Here's how the part is built. I have some questions about the finished solid (model axes, mm). Face numbers are marked on the shaded views. Coordinates: 2 decimals unless noted, no trailing zeros. Loops run counter-clockwise (first coordinate to the right, second up) from the corner with the lowest first, then second, coordinate; pieces in that order, holes last. Notation, with made-up numbers: (41.25, 38.5) - (48.25, 38.5) arc R22 ccw to (48.25, 55.5) - close; hole circle Ø6 at (53, -36.75). An arc over 180 degrees is marked (long way). Use a Markdown table: item, result.
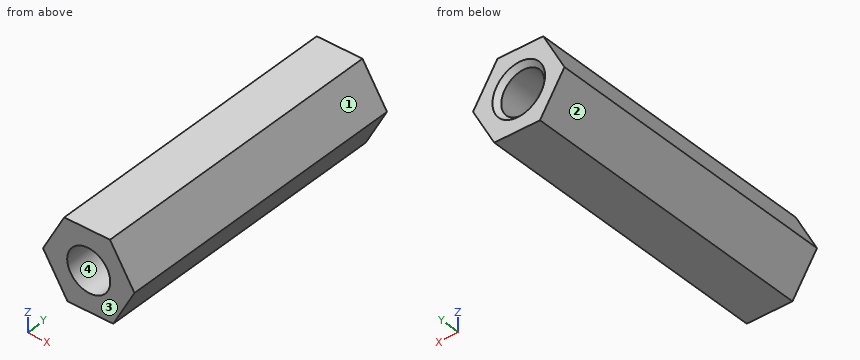
```python
from build123d import *

# Parameters (mm, degrees)
SKETCH_1_R                   = 1.1
EXTRUDE_1_DEPTH              = 17
HOLE_WIZARD_M3_2_D           = 2.5
HOLE_WIZARD_M3_2_CSINK_D     = 3.05
HOLE_WIZARD_M3_2_CSINK_ANGLE = 90


with BuildPart() as part:
    # 草图1 → 凸台-拉伸1 (new body)
    with BuildSketch(Plane(origin=(0, 0, 0), x_dir=(1, 0, 0), z_dir=(0, 1, 0))):
        Polygon((1.231724884, -2.352910356), (2.653542583, -0.109750138), (1.421817699, 2.243160218), (-1.231724884, 2.352910356), (-2.653542583, 0.109750138), (-1.421817699, -2.243160218), align=None)
        Circle(SKETCH_1_R, mode=Mode.SUBTRACT)
    extrude(amount=EXTRUDE_1_DEPTH)

    # M3 螺纹孔2 (through all)
    with Locations(Plane(origin=(0, 17, 0), x_dir=(1, 0, 0), z_dir=(0, 1, 0))):
        with Locations((0, 0)):
            CounterSinkHole(HOLE_WIZARD_M3_2_D / 2, HOLE_WIZARD_M3_2_CSINK_D / 2, counter_sink_angle=HOLE_WIZARD_M3_2_CSINK_ANGLE)


solid = part.part
```
Q1. I want a section at A-A, the plane y = 13.75. Write out the boundary of the cut face in (x, z).
Check values:
| item | result |
|---|---|
| outline | (-2.65, -0.11) - (-1.23, -2.35) - (1.42, -2.24) - (2.65, 0.11) - (1.23, 2.35) - (-1.42, 2.24) - close; hole circle Ø2.5 at (0, 0) |
Q2. I want a section at C-C, the plane z = 1.7. Write out the boundary of the cut face in (x, y), then the cut area to 3 significant figures.
Check values:
| item | result |
|---|---|
| outline | (-1.71, 0) - (1.65, 0) - (1.65, 17) - (-1.71, 17) - close |
| area | 57.0 mm^2 |
Q3. Please list where these lines run through material, in increasing order: L1, parallel to Z at x = 0.6, y = 6; L2, parallel to X at y = 16.25, z = -0.9; L3, parallel to Z at x = 0.2, y = 16.25. Write a range as from..to.
Check values:
| item | result |
|---|---|
| L1 | -2.28..-1.1, 1.1..2.33 |
| L2 | -2.15..-0.87, 0.87..2.12 |
| L3 | -2.29..-1.23, 1.23..2.31 |
Q4. If we mould it in two halves opening along Z, with no side actions, what happens to the marked faces 1, 2, 3 and 4? For each: pulls with the +Z half, pulls with the -Z half, needs draft (parallel to the pull), parting line crosses it, or undercut.
Check values:
| item | result |
|---|---|
| face 1 | pulls with the +Z half |
| face 2 | pulls with the -Z half |
| face 3 | needs draft |
| face 4 | undercut |
Q5. I want a section at D-D, the plane x = -2. Write out the boundary of the cut face in (y, z), then the cut area to 3 significant figures.
Check values:
| item | result |
|---|---|
| outline | (0, -1.14) - (17, -1.14) - (17, 1.14) - (0, 1.14) - close |
| area | 38.8 mm^2 |
Q6. Will these pins go through, and if not, where does the flat tip stop? P1, Ø2, axis at x = 1.5, y = 12, coming from the +Z side; P2, Ø1, axis at x = 0, y = 3, coming from the +Z side.
Check values:
| item | result |
|---|---|
| P1 | z = 2.35 |
| P2 | z = 2.32 |
Q7. I want a section at B-B, the plane x = 0. Write out the boundary of the cut face in (y, z) (3 decimals).
Check values:
| item | result |
|---|---|
| outline | (0, -2.302) - (17, -2.302) - (17, -1.525) - (16.725, -1.25) - (0, -1.25) - close; (0, 1.25) - (16.725, 1.25) - (17, 1.525) - (17, 2.302) - (0, 2.302) - close |
